Design review of the part built by this model. Coordinates are the model's own, in mm. Face numbers are marked on the shaded views. A direction names the side the tool comes from. Coordinates: 2 decimals unless noted, no trailing zeros. Order: outer loops, then holes, each group sorted by start corner. A loop starts at its lowest first (then second) coordinate and runs counter-clockwise, first axis right, second up. Notation, with made-up numbers: (-10.5, -0.75) -> (14.5, -0.75) arc R26 ccw to (14.5, 25.25) -> close; hole circle Ø5 at (40, 47). An arc over 180 degrees is marked (long way). Use a Markdown table: item, result. Add a question column.
Q1. Insertion check: pin 1 (4.5 mm diameter, centred on x = -5, y = -12, fed in from +Z); pin 2 (2 mm diameter, centred on y = -4, z = 2.5, fed in from +X); pin 3 (4 mm diameter, centred on x = -0.5, y = -3.5, fed in from +Z). Each pin has a flat end and moves straight along its axis. Give the tip position at first contact, or say it passes through.
Q2. The part is to be moulded in two halves that separate along X. For the marked faces 1, 2 and 3, say which applies: pulls with the +X half, pulls with the -X half, needs draft (parallel to the pull), parting line crosses it, or undercut.
Q3. Machinability: for the marked faces 4, 5, 6 and 7, which of the approach directions +Z, -Z, +X, -X, +Y, -Y give a long, thin tool a straight path to every point of the face, cutting with its end or side? Answer none if there is none.
Q4. Add section C-C (y = 0). State the section outline as (x, z) points.
Q5. Add section A-A (x = -3.76). State the section outline as (y, z) points, then the cut area to 3 significant figures.
Q6. Add section B-B (z = 2). Count the separate pieces of the cut face and the enclosed holes in it, then the cut area to 3 significant figures.
Q7. Wall thickness on probe 1 along Y at (x, z) = (-3.76, 0.35); probe 2 along Z at (x, y) = (-6.25, -10.5); probe 3 along Y at (x, z) = (-5, 2): over which ranges is each line inside the solid? List them lowest first.
Solid Edge part; units mm, degrees
sketch "Sketch1" plane through (0, 0, 0) normal (1, 0, 0) x (0, 1, 0)
  line L0 (6.5, 0) -> (15.52, 0)
  line L1 (15.52, 0) -> (15.52, 4)
  line L2 (15.52, 4) -> (6.3443, 4)
  line L3 (-15.52, 4) -> (-6.3443, 4)
  line L4 (-15.52, 0) -> (-15.52, 4)
  line L5 (-6.5, 0) -> (-15.52, 0)
  arc A0 (-6.5, 0) -> (6.5, 0) centre (0, 0) cw
  arc A1 (6.3443, 4) -> (-6.3443, 4) centre (0, 0) ccw
  dimension "D1" = 6.5
  dimension "D2" = 15.52
  dimension "D3" = 15.52
  dimension "D4" = 15.52
extrude "Protrusion1" add sketch "Sketch1" against normal blind 7.52
hole "Bohrung_1" at (-3.76, 11.01, 4) direction (0, 0, -1) diameter 2.7 end through all counterbore diameter 5.5 counterbore depth 3
mirror "Mirror1" about plane through (0, 0, 0) normal (0, -1, 0) of "Bohrung_1"
sketch "Sketch2" plane through (0, 0, 3.75) normal (1, 0, 0) x (0, 1, 0)
  line L0 (-6.5, -3.75) -> (-4, -3.75)
  line L1 (4, -3.75) -> (6.5, -3.75)
  arc A0 (-4, -3.75) -> (4, -3.75) centre (0, -3.75) cw
  arc A1 (6.5, -3.75) -> (-6.5, -3.75) centre (0, -3.75) ccw
extrude "Extrusionsausprägung_2" add sketch "Sketch2" against normal blind 1.52
sketch "Sketch3" plane through (-7.52, 0, 3.75) normal (-1, 0, 0) x (0, -1, 0)
  line L0 (-6.5, -3.75) -> (-5.5, -3.75)
  line L1 (5.5, -3.75) -> (6.5, -3.75)
  arc A0 (-5.5, -3.75) -> (5.5, -3.75) centre (0, -3.75) cw
  arc A1 (6.5, -3.75) -> (-6.5, -3.75) centre (0, -3.75) ccw
extrude "Extrusionsausprägung_3" add sketch "Sketch3" against normal blind 1
sketch "Sketch4" plane through (-3.76, 12.52, 2) normal (0, 1, 0) x (-1, 0, 0)
  line L0 (-3.76, 2) -> (-4.76, 2)
  line L1 (-4.76, 2) -> (-4.76, -2)
  line L2 (-4.76, -2) -> (-3.76, -2)
  line L3 (-3.76, -2) -> (-3.76, 2)
  dimension "D1" = 3.76
extrude "Extrusionsausprägung_4" add sketch "Sketch4" against normal blind 2
fillet "Verrundung_1" radius 1 3 edges at (1, 11.52, 4) (1, 12.52, 2) (1, 10.52, 2)
mirror "Mirror2" about plane through (0, 0, 0) normal (0, -1, 0) of "Extrusionsausprägung_4"
fillet "Round1" radius 1 3 edges at (1, -11.52, 4) (1, -12.52, 2) (1, -10.52, 2)
properties material "Plastic ABS (extra strong)"
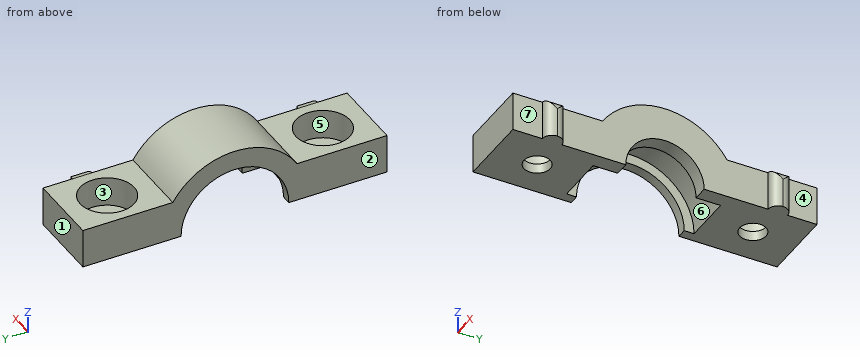
Established:
| question | item | result |
|---|---|---|
| 1 | pin 1 | z = 4 |
| 1 | pin 2 | x = 0 |
| 1 | pin 3 | z = 7.35 |
| 2 | face 1 | needs draft |
| 2 | face 2 | pulls with the -X half |
| 2 | face 3 | undercut |
| 3 | face 4 | +Z, -Z, +X, +Y |
| 3 | face 5 | +Z |
| 3 | face 6 | -Z |
| 3 | face 7 | +Z, -Z, +X, -Y |
| 4 | outline | (-7.52, 5.5) -> (-6.52, 5.5) -> (-6.52, 6.5) -> (-1.52, 6.5) -> (-1.52, 4) -> (0, 4) -> (0, 7.5) -> (-7.52, 7.5) -> close |
| 5 | outline | (-15.52, 0) -> (-12.36, 0) -> (-12.36, 1) -> (-13.76, 1) -> (-13.76, 4) -> (-15.52, 4) -> close; (-9.66, 0) -> (-6.5, 0) arc R6.5 cw to (6.5, 0) -> (9.66, 0) -> (9.66, 1) -> (8.26, 1) -> (8.26, 4) -> (6.34, 4) arc R7.5 ccw to (-6.34, 4) -> (-8.26, 4) -> (-8.26, 1) -> (-9.66, 1) -> close; (12.36, 0) -> (15.52, 0) -> (15.52, 4) -> (13.76, 4) -> (13.76, 1) -> (12.36, 1) -> close |
| 5 | area | 50.7 mm^2 |
| 6 | separate pieces | 2 |
| 6 | enclosed holes | 2 |
| 6 | area | 106 mm^2 |
| 7 | probe 1 | -15.52 to -12.36, -9.66 to -6.49, 6.49 to 9.66, 12.36 to 15.52 |
| 7 | probe 2 | 0 to 1 |
| 7 | probe 3 | -15.52 to -13.46, -8.56 to -6.18, 6.18 to 8.56, 13.46 to 15.52 |
